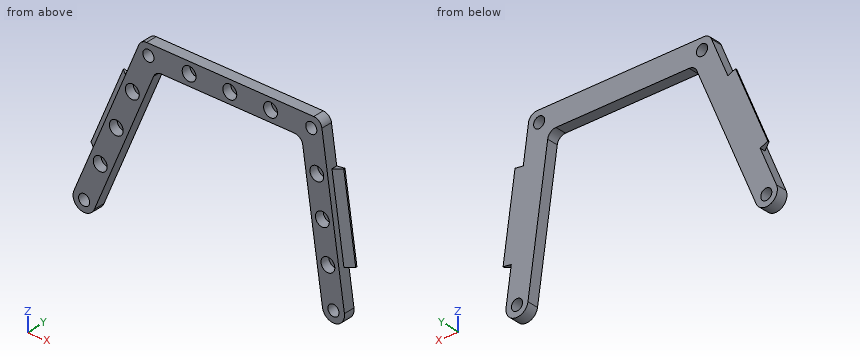
from build123d import *

# Parameters (mm, degrees)
BOSS_EXTRUDE1_DEPTH = 4
SKETCH5_R           = 2.5
CUT_EXTRUDE1_DEPTH  = 3.25
SKETCH6_W           = 30
SKETCH6_H           = 0.5
BOSS_EXTRUDE2_DEPTH = 3
BOSS_EXTRUDE3_DEPTH = 30
SKETCH8_W           = 30
SKETCH8_H           = 0.5
BOSS_EXTRUDE4_DEPTH = 3
BOSS_EXTRUDE5_DEPTH = 30
SKETCH10_R          = 2
CUT_EXTRUDE2_DEPTH  = 4


# Read off the part's stored shape, not the designer's step: M3x0.5 Tapped Hole1
with BuildPart() as part:
    # Sketch1 → Boss-Extrude1 (new body)
    with BuildSketch(Plane(origin=(0, 0, 0), x_dir=(1, 0, 0), z_dir=(0, 1, 0))):
        with BuildLine():
            Line((-26.885531635, 53.445375747), (-3.427655647, -2.16596819))
            ThreePointArc((-3.427655647, -2.16596819), (-2.322135184, -3.499790448), (-0.663506921, -4))
            Line((-0.663506921, -4), (59.665068599, -4))
            ThreePointArc((59.665068599, -4), (61.627788827, -3.268860795), (62.633827917, -1.431819537))
            Line((62.633827917, -1.431819537), (70.758345757, 54.424240617))
            ThreePointArc((70.758345757, 54.424240617), (67.375759383, 58.958345757), (62.841654243, 55.575759383))
            Line((62.841654243, 55.575759383), (55.713279127, 6.568180463))
            ThreePointArc((55.713279127, 6.568180463), (54.707240038, 4.731139205), (52.744519809, 4))
            Line((52.744519809, 4), (4.644548446, 4))
            ThreePointArc((4.644548446, 4), (2.985920183, 4.500209552), (1.88039972, 5.83403181))
            Line((1.88039972, 5.83403181), (-19.514468365, 56.554624253))
            ThreePointArc((-19.514468365, 56.554624253), (-24.754624253, 58.685531635), (-26.885531635, 53.445375747))
        make_face()
    extrude(amount=BOSS_EXTRUDE1_DEPTH)

    # M3x0.5 Tapped Hole1 outline → M3x0.5 Tapped Hole1 (revolve, cut)
    with BuildSketch(Plane(origin=(-23.2, 0, -55), x_dir=(1, 0, 0), z_dir=(0, 0, 1))):
        Polygon((0, 0), (1.25, 0), (1.25, 3.725), (1.525, 4), (0, 4), align=None)
    revolve(axis=Axis((-23.2, 0, -55), (0, 1, 0)), mode=Mode.SUBTRACT)

    # M3x0.5 Tapped Hole1 2 outline → M3x0.5 Tapped Hole1 2 (revolve, cut)
    with BuildSketch(Plane.XY):
        Polygon((0, 0), (1.25, 0), (1.25, 3.725), (1.525, 4), (0, 4), align=None)
    revolve(axis=Axis((0, 0, 0), (0, 1, 0)), mode=Mode.SUBTRACT)

    # M3x0.5 Tapped Hole1 3 outline → M3x0.5 Tapped Hole1 3 (revolve, cut)
    with BuildSketch(Plane(origin=(58.8, 0, 0), x_dir=(1, 0, 0), z_dir=(0, 0, 1))):
        Polygon((0, 0), (1.25, 0), (1.25, 3.725), (1.525, 4), (0, 4), align=None)
    revolve(axis=Axis((58.8, 0, 0), (0, 1, 0)), mode=Mode.SUBTRACT)

    # M3x0.5 Tapped Hole1 4 outline → M3x0.5 Tapped Hole1 4 (revolve, cut)
    with BuildSketch(Plane(origin=(66.8, 0, -55), x_dir=(1, 0, 0), z_dir=(0, 0, 1))):
        Polygon((0, 0), (1.25, 0), (1.25, 3.725), (1.525, 4), (0, 4), align=None)
    revolve(axis=Axis((66.8, 0, -55), (0, 1, 0)), mode=Mode.SUBTRACT)

    # Sketch5 → Cut-Extrude1 (cut)
    with BuildSketch(Plane.XZ):
        with Locations(Location((-17.4, -41.25, 0), (0, 0, 270))):
            Circle(SKETCH5_R)
        with Locations(Location((29.4, 0, 0), (0, 0, 270))):
            Circle(SKETCH5_R)
        with Locations(Location((60.8, -13.75, 0), (0, 0, 270))):
            Circle(SKETCH5_R)
        with Locations(Location((-5.8, -13.75, 0), (0, 0, 270))):
            Circle(SKETCH5_R)
        with Locations(Location((64.8, -41.25, 0), (0, 0, 270))):
            Circle(SKETCH5_R)
        with Locations(Location((-11.6, -27.5, 0), (0, 0, 270))):
            Circle(SKETCH5_R)
        with Locations(Location((14.7, 0, 0), (0, 0, 270))):
            Circle(SKETCH5_R)
        with Locations(Location((44.1, 0, 0), (0, 0, 270))):
            Circle(SKETCH5_R)
        with Locations(Location((62.8, -27.5, 0), (0, 0, 270))):
            Circle(SKETCH5_R)
    extrude(amount=-CUT_EXTRUDE1_DEPTH, mode=Mode.SUBTRACT)

    # Sketch6 → Boss-Extrude2 (add)
    with BuildSketch(Plane(origin=(-3.685531635, 0, 1.554624253), x_dir=(0.38865606330829405, 0, 0.921382908705007), z_dir=(-0.921382908705007, 0, 0.38865606330829405))):
        with Locations((-29.514686863, 3.75)):
            Rectangle(SKETCH6_W, SKETCH6_H)
    extrude(amount=BOSS_EXTRUDE2_DEPTH)

    # Sketch7 → Boss-Extrude3 (add)
    with BuildSketch(Plane(origin=(-5.641221056, 0, -13.373584401), x_dir=(0.9213829087050069, 0, -0.3886560633082941), z_dir=(0.3886560633082942, 0, 0.921382908705007))):
        Polygon((-4, 2), (-4, 3.5), (-7, 3.5), align=None)
    extrude(amount=-BOSS_EXTRUDE3_DEPTH)

    # Sketch8 → Boss-Extrude4 (add)
    with BuildSketch(Plane(origin=(61.540087421, 0, 8.951285443), x_dir=(0.14393984571411056, 0, -0.9895864392845114), z_dir=(0.9895864392845114, 0, 0.14393984571411056))):
        with Locations((35.820515092, 3.75)):
            Rectangle(SKETCH8_W, SKETCH8_H)
    extrude(amount=BOSS_EXTRUDE4_DEPTH)

    # Sketch9 → Boss-Extrude5 (add)
    with BuildSketch(Plane(origin=(2.99690173, 0, -20.603699394), x_dir=(0.9895864392845114, 0, 0.14393984571411056), z_dir=(-0.14393984571411056, 0, 0.9895864392845114))):
        Polygon((65.18768263, 3.5), (62.18768263, 3.5), (62.18768263, 2), align=None)
    extrude(amount=-BOSS_EXTRUDE5_DEPTH)

    # Sketch10 → Cut-Extrude2 (cut)
    with BuildSketch(Plane(origin=(0, 4, 0), x_dir=(1, 0, 0), z_dir=(0, 1, 0))):
        with Locations(Location((-23.2, 55, 0), (0, 0, 270))):
            Circle(SKETCH10_R)
        with Locations(Location((0, 0, 0), (0, 0, 270))):
            Circle(SKETCH10_R)
        with Locations(Location((58.8, 0, 0), (0, 0, 270))):
            Circle(SKETCH10_R)
        with Locations(Location((66.8, 55, 0), (0, 0, 270))):
            Circle(SKETCH10_R)
    extrude(amount=-CUT_EXTRUDE2_DEPTH, mode=Mode.SUBTRACT)


solid = part.part
Work out the finished part from the listing and answer in its coordinate system (mm). Round coordinates to 2 decimals unless told otherwise and drop trailing zeros. Loops run counter-clockwise (first coordinate to the right, second up) from the corner with the lowest first, then second, coordinate; pieces in that order, holes last. Notation, with made-up numbers: (15.25, -35) - (20.25, -35) arc R4 cw to (20.25, -31) - close; hole circle Ø4 at (-16.5, 47). An arc over 180 degrees is marked (long way). One line per item, written item: value.
Q1. Find section C-C on z = 0. Give the vertices of the cut face in (x, y).
Check values:
outline: (-4.34, 0) - (-2, 0) - (-2, 4) - (-4.34, 4) - close; (2, 0) - (12.2, 0) - (12.2, 3.25) - (17.2, 3.25) - (17.2, 0) - (26.9, 0) - (26.9, 3.25) - (31.9, 3.25) - (31.9, 0) - (41.6, 0) - (41.6, 3.25) - (46.6, 3.25) - (46.6, 0) - (56.8, 0) - (56.8, 4) - (2, 4) - close; (60.8, 0) - (62.84, 0) - (62.84, 4) - (60.8, 4) - close
Q2. Find section B-B on y = 0.7. State how many separate pieces and enclosed holes the cut face has, and give its area (3 significant figures).
Check values:
separate pieces: 1
enclosed holes: 13
area: 1,220 mm2
Q3. Each of these flat-tipped pins is pushed along its axis until it touches: pin 1 Ø2.5 at (x, z) = (64.5, -42) entering from -Y; pin 2 Ø8 at (x, z) = (-17.4, -41.25) entering from -Y; pin 3 Ø1.5 at (y, z) = (3, -20) entering from +X; pin 4 Ø1.5 at (y, z) = (0.5, -7) entering from +X. Where does it stop, or does it pass through?
Check values:
pin 1: y = 3.25
pin 2: y = 0
pin 3: x = 68.86
pin 4: x = 63.97
Q4. Find section A-A on x = 29.4. Give the vertices of the cut face in (y, z), and give its area (4 significant figures).
Check values:
outline: (0, -4) - (4, -4) - (4, 4) - (0, 4) - (0, 2.5) - (3.25, 2.5) - (3.25, -2.5) - (0, -2.5) - close
area: 15.75 mm2
Q5. Straight lines are drawn through the part: probe 1 along X at (y, z) = (0.7, -27.5); probe 2 along X at (y, z) = (2.55, -12); probe 3 along X at (y, z) = (2.35, 0). For each, find the intervals that lie inside material, in ascending order.
Check values:
probe 1: -15.94 to -14.1, -9.1 to -7.26, 58.76 to 60.3, 65.3 to 66.84
probe 2: -10.6 to -7.59, -4.01 to -0.72, 56.5 to 59.01, 62.59 to 65.7
probe 3: -4.34 to -2, 2 to 12.2, 17.2 to 26.9, 31.9 to 41.6, 46.6 to 56.8, 60.8 to 62.84
Q6. Find section D-D on z = -36. Give the vertices of the cut face in (x, y).
Check values:
outline: (-22.78, 3.5) - (-19.53, 2) - (-19.53, 0) - (-10.84, 0) - (-10.84, 4) - (-22.78, 4) - close; (59.99, 0) - (68.08, 0) - (68.08, 2) - (71.11, 3.5) - (71.11, 4) - (59.99, 4) - close
